```python
from build123d import *

# Parameters (mm, degrees)
F0_R     = 24.5
F0_R_2   = 7.5
F1_DEPTH = 10


with BuildPart() as f1:
    # F0 (on Top) → F1 (new body)
    with BuildSketch(Plane.XY):
        Circle(F0_R)
        with BuildLine():
            Line((0, -11.500001), (0, -20.500001))
            ThreePointArc((0, -20.500001), (-7.845011, -18.939531), (-14.49569, -14.49569))
            Line((-14.49569, -14.49569), (-8.131729, -8.131729))
            ThreePointArc((-8.131729, -8.131729), (-4.40086, -10.624615), (0, -11.500001))
        make_face(mode=Mode.SUBTRACT)
        with BuildLine():
            Line((-9.959293, -5.75), (-17.753521, -10.25))
            ThreePointArc((-17.753521, -10.25), (-20.32462, -2.675787), (-19.80148, 5.30579))
            Line((-19.80148, 5.30579), (-11.108148, 2.976419))
            ThreePointArc((-11.108148, 2.976419), (-11.401617, -1.501052), (-9.959293, -5.75))
        make_face(mode=Mode.SUBTRACT)
        Circle(F0_R_2, mode=Mode.SUBTRACT)
        with BuildLine():
            Line((9.959292, -5.750001), (17.753521, -10.250001))
            ThreePointArc((17.753521, -10.250001), (12.479609, -16.263744), (5.30579, -19.80148))
            Line((5.30579, -19.80148), (2.976419, -11.108148))
            ThreePointArc((2.976419, -11.108148), (7.000756, -9.123564), (9.959292, -5.750001))
        make_face(mode=Mode.SUBTRACT)
        with BuildLine():
            Line((-9.959293, 5.75), (-17.753521, 10.25))
            ThreePointArc((-17.753521, 10.25), (-12.47961, 16.263744), (-5.305791, 19.801479))
            Line((-5.305791, 19.801479), (-2.976419, 11.108147))
            ThreePointArc((-2.976419, 11.108147), (-7.000757, 9.123563), (-9.959293, 5.75))
        make_face(mode=Mode.SUBTRACT)
        with BuildLine():
            Line((9.959292, 5.75), (17.753521, 10.25))
            ThreePointArc((17.753521, 10.25), (20.32462, 2.675786), (19.80148, -5.305791))
            Line((19.80148, -5.305791), (11.108147, -2.97642))
            ThreePointArc((11.108147, -2.97642), (11.401616, 1.501051), (9.959292, 5.75))
        make_face(mode=Mode.SUBTRACT)
        with BuildLine():
            Line((0, 11.5), (0, 20.5))
            ThreePointArc((0, 20.5), (7.845011, 18.93953), (14.495689, 14.495689))
            Line((14.495689, 14.495689), (8.131728, 8.131728))
            ThreePointArc((8.131728, 8.131728), (4.40086, 10.624615), (0, 11.5))
        make_face(mode=Mode.SUBTRACT)
    extrude(amount=F1_DEPTH)


solid = f1.part
```
Check sheet for the modelled part. Datum: model origin and axes. Units: mm. Give positions to 0.01 mm unless a question says otherwise; leave off trailing zeros. Write each loop counter-clockwise with the first axis right and the second up, starting at its lowest first coordinate (ties: lowest second). Pieces come first, ordered by that corner, then holes. Notation, with made-up numbers: (22, -11.75) - (48, -11.75) arc R22 ccw to (48, 0.25) - close; hole circle Ø8 at (37.5, 16.25). An arc over 180 degrees is marked (long way). Answer as a JSON object with one key per item and string values. Group by question number.
1) Sectioned sample at D-D (y = 18.5). Record the cut outline in (x, z).
2) Release check for a two-part mould opening along X. For faces 1 (the face through (13.17, 20.66, 4.93)), 2 (the face through (-4.46, -10.6, 4.93)), 3 (the face through (-6, -5, 10)) record: pulls with the +X half, pulls with the -X half, needs draft (parallel to the pull), parting line crosses it, or undercut.
3) Thickness scan on probe 1 along X at (y, z) = (-2, 9.75); probe 2 along Y at (x, z) = (-9, 2.5); probe 3 along X at (y, z) = (-15, 1.5). Record the ranges inside material, lowest first. Write a range as from..to.
4) Depth check by flat-ended pin: P1, Ø1, axis at x = -4, z = 5, coming from the -Y side; P2, Ø1, axis at y = 12, z = 5.5, coming from the +X side; P3, Ø12, axis at x = 0, y = 0, coming from the +Z side; P4, Ø4.5, axis at y = -14.5, z = 4.5, coming from the -X side. Enter the tip coordinate at first touch or a pass-through.
5) Sectioned sample at B-B (z = 1). Record the cut outline in (x, y).
6) Sectioned sample at C-C (x = -18.5). Record the cut outline in (y, z), then the cut area to 3 significant figures.
7) Sectioned sample at A-A (y = 0). Record the cut outline in (x, z), then the cut area to 3 significant figures.
Geometry results:
{
 "1": {"outline": "(-16.06, 0) - (-8.83, 0) - (-8.83, 10) - (-16.06, 10) - close; (-4.96, 0) - (0, 0) - (0, 10) - (-4.96, 10) - close; (8.83, 0) - (16.06, 0) - (16.06, 10) - (8.83, 10) - close"},
 "2": {"face 1": "parting line crosses it", "face 2": "undercut", "face 3": "needs draft"},
 "3": {"probe 1": "x = -24.42..-20.4, -11.32..-7.23, 7.23..11.32, 20.4..24.42", "probe 2": "y = -22.79..-18.42, -9..7.16, 18.42..22.79", "probe 3": "x = -19.37..-13.97, 0..4.02, 13.97..19.37"},
 "4": {"P1": "stops at y = -24.25", "P2": "stops at x = 21.63", "P3": "passes through", "P4": "stops at x = -21.22"},
 "5": {"outline": "circle Ø49 at (0, 0); hole (-19.8, 5.31) arc R20.5 ccw to (-17.75, -10.25) - (-9.96, -5.75) arc R11.5 cw to (-11.11, 2.98) - close; hole (-17.75, 10.25) - (-9.96, 5.75) arc R11.5 cw to (-2.98, 11.11) - (-5.31, 19.8) arc R20.5 ccw to start; hole (-14.5, -14.5) arc R20.5 ccw to (0, -20.5) - (0, -11.5) arc R11.5 cw to (-8.13, -8.13) - close; hole circle Ø15 at (0, 0); hole (0, 11.5) arc R11.5 cw to (8.13, 8.13) - (14.5, 14.5) arc R20.5 ccw to (0, 20.5) - close; hole (2.98, -11.11) - (5.31, -19.8) arc R20.5 ccw to (17.75, -10.25) - (9.96, -5.75) arc R11.5 cw to start; hole (9.96, 5.75) arc R11.5 cw to (11.11, -2.98) - (19.8, -5.31) arc R20.5 ccw to (17.75, 10.25) - close"},
 "6": {"outline": "(-16.06, 0) - (-8.83, 0) - (-8.83, 10) - (-16.06, 10) - close; (4.96, 0) - (16.06, 0) - (16.06, 10) - (4.96, 10) - close", "area": "183 mm^2"},
 "7": {"outline": "(-24.5, 0) - (-20.5, 0) - (-20.5, 10) - (-24.5, 10) - close; (-11.5, 0) - (-7.5, 0) - (-7.5, 10) - (-11.5, 10) - close; (7.5, 0) - (11.5, 0) - (11.5, 10) - (7.5, 10) - close; (20.5, 0) - (24.5, 0) - (24.5, 10) - (20.5, 10) - close", "area": "160 mm^2"}
}
